```python
from build123d import *

# Parameters (mm, degrees)
F0_W     = 152.4
F0_H     = 20.3
F0_W_2   = 33
F0_H_2   = 14
F1_DEPTH = 8.6
F2_W     = 152.4
F2_H     = 13.6
F3_DEPTH = 4.6
F6_DEPTH = 8.6
F7_W     = 27
F7_H     = 25
F8_DEPTH = 2
F4_R     = 0.75
F9_DEPTH = 4.001


with BuildPart() as f1:
    # F0 (on Top) → F1 (new body)
    with BuildSketch(Plane.XY):
        Rectangle(F0_W, F0_H)
        with Locations((-43.375, 0)):
            Rectangle(F0_W_2, F0_H_2, mode=Mode.SUBTRACT)
        with Locations((43.375, 0)):
            Rectangle(F0_W_2, F0_H_2, mode=Mode.SUBTRACT)
    extrude(amount=F1_DEPTH)

    # F2 (on face) → F3 (cut)
    with BuildSketch(Plane.XY.offset(8.6)):
        Rectangle(F2_W, F2_H)
    extrude(amount=-F3_DEPTH, mode=Mode.SUBTRACT)

    # F5 (on face) → F6 (join, through all)
    with BuildSketch(Plane.XY.offset(8.6)):
        with BuildLine():
            Line((7, 15.8900657923), (7, 10.15))
            Line((7, 10.15), (30, 10.15))
            Line((30, 10.15), (30, 15.8900657923))
            ThreePointArc((30, 15.8900657923), (29.45, 16.65), (30, 17.4099342077))
            Line((30, 17.4099342077), (30, 25.8900657923))
            ThreePointArc((30, 25.8900657923), (29.45, 26.65), (30, 27.4099342077))
            Line((30, 27.4099342077), (30, 33.15))
            Line((30, 33.15), (7, 33.15))
            Line((7, 33.15), (7, 27.4099342077))
            ThreePointArc((7, 27.4099342077), (7.3980740698, 27.119041576), (7.55, 26.65))
            ThreePointArc((7.55, 26.65), (7.3980740698, 26.180958424), (7, 25.8900657923))
            Line((7, 25.8900657923), (7, 17.4099342077))
            ThreePointArc((7, 17.4099342077), (7.3980740698, 17.119041576), (7.55, 16.65))
            ThreePointArc((7.55, 16.65), (7.3980740698, 16.180958424), (7, 15.8900657923))
        make_face()
        with BuildLine():
            Line((5, 10.15), (7, 10.15))
            Line((7, 10.15), (7, 15.8900657923))
            ThreePointArc((7, 15.8900657923), (5.95, 16.65), (7, 17.4099342077))
            Line((7, 17.4099342077), (7, 25.8900657923))
            ThreePointArc((7, 25.8900657923), (5.95, 26.65), (7, 27.4099342077))
            Line((7, 27.4099342077), (7, 33.15))
            Line((7, 33.15), (30, 33.15))
            Line((30, 33.15), (30, 27.4099342077))
            ThreePointArc((30, 27.4099342077), (30.719041576, 27.2980740698), (31.05, 26.65))
            ThreePointArc((31.05, 26.65), (30.719041576, 26.0019259302), (30, 25.8900657923))
            Line((30, 25.8900657923), (30, 17.4099342077))
            ThreePointArc((30, 17.4099342077), (30.719041576, 17.2980740698), (31.05, 16.65))
            ThreePointArc((31.05, 16.65), (30.719041576, 16.0019259302), (30, 15.8900657923))
            Line((30, 15.8900657923), (30, 10.15))
            Line((30, 10.15), (32, 10.15))
            Line((32, 10.15), (32, 35.15))
            Line((32, 35.15), (5, 35.15))
            Line((5, 35.15), (5, 10.15))
        make_face()
    extrude(amount=-F6_DEPTH)

    # F7 (on face) → F8 (cut)
    with BuildSketch(Plane.XY.offset(8.6)):
        with Locations((18.5, 22.65)):
            Rectangle(F7_W, F7_H)
    extrude(amount=-F8_DEPTH, mode=Mode.SUBTRACT)

    # F4 (on face) → F9 (cut, through all)
    with BuildSketch(Plane.XY.offset(4)):
        with Locations((24, 3)):
            Circle(F4_R)
        with Locations((-25, -3)):
            Circle(F4_R)
        with Locations((-65, 3)):
            Circle(F4_R)
        with Locations((69, -3)):
            Circle(F4_R)
    extrude(amount=-F9_DEPTH, mode=Mode.SUBTRACT)


solid = f1.part
```
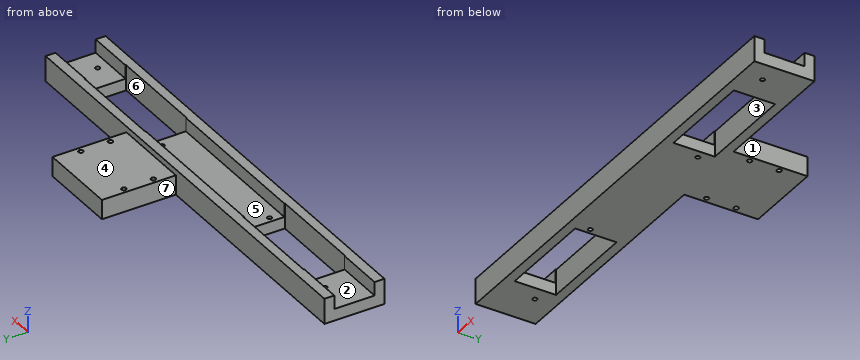
Could you check a few things on this model? Use its own coordinates, in mm. Face numbers are marked on the shaded views. A direction names the side the tool comes from. Coordinates: 2 decimals unless noted, no trailing zeros. Write each loop counter-clockwise with the first axis right and the second up, starting at its lowest first coordinate (ties: lowest second). Pieces come first, ordered by that corner, then holes. Notation, with made-up numbers: (58, 17.25) -> (82, 17.25) arc R19 ccw to (82, 29.25) -> close; hole circle Ø3 at (27.5, 77). An arc over 180 degrees is marked (long way). Write item = value, one per line. Start each with the question number.
(1) Which directions (+Z, -Z, +X, -X, +Y, -Y) give clear straight access to the entire face, cutting with the end or side of a thin tool? Please do the marked faces 4, 5, 6 and 7.
(2) I want a section at B-B (x = -51). Please give me the cut outline in (y, z).
(3) I want a section at A-A (z = 1.5). Give the number of separate pieces and of enclosed holes in the cut face, plus the area to 3 significant figures.
(4) Will these pins go through, and if not, where does the flat tip stop? pin 1 (2.5 mm diameter, centred on x = 6.75, y = 16.65, fed in from +Z); pin 2 (6 mm diameter, centred on x = -15.5, y = 0, fed in from +Z); pin 3 (2.5 mm diameter, centred on x = 66.5, z = 5.5, fed in from +Y).
(5) We'd pull the mould along X, two halves only. Please class the marked faces 1, 2 and 3: released by +X, released by -X, zero draft, split by the parting line, or undercut.
(6) I want a section at C-C (y = 24). Please give me the cut outline in (x, z).
(7) I want a section at D-D (x = 66). Please give me the cut outline in (y, z), plus the area to 3 significant figures.
(8) I need wall thicknesses on line 1 (Y direction, x = 6.75, z = 2.5); line 2 (Y direction, x = 54, z = 8); line 3 (Y direction, x = 29, z = 6.5). Which ranges of each line are inside material? Lowest first, please. Write a range as [from, to].
Result set:
q1.face_4 = +Z, +X, -X, +Y
q1.face_5 = +Z, +X, -X
q1.face_6 = +Z, -Z
q1.face_7 = +Z, -Z, -X, +Y
q2.outline = (-10.15, 0) -> (-7, 0) -> (-7, 8.6) -> (-10.15, 8.6) -> close; (7, 0) -> (10.15, 0) -> (10.15, 8.6) -> (7, 8.6) -> close
q3.separate_pieces = 1
q3.enclosed_holes = 10
q3.area = 2,830 mm2
q4.pin_1 = 6.6
q4.pin_2 = 4
q4.pin_3 = 10.15
q5.face_1 = released by +X
q5.face_2 = zero draft
q5.face_3 = undercut
q6.outline = (5, 0) -> (32, 0) -> (32, 6.6) -> (5, 6.6) -> close
q7.outline = (-10.15, 0) -> (10.15, 0) -> (10.15, 8.6) -> (6.8, 8.6) -> (6.8, 4) -> (-6.8, 4) -> (-6.8, 8.6) -> (-10.15, 8.6) -> close
q7.area = 112 mm2
q8.line_1 = [-10.15, 15.85], [17.45, 25.85], [27.45, 35.15]
q8.line_2 = [-10.15, -7], [7, 10.15]
q8.line_3 = [-10.15, -7], [7, 35.15]
